```python
from build123d import *

# Parameters (mm, degrees)
F0_W          = 60
F0_H          = 60
F0_R          = 3.5
F1_DEPTH      = 8
F1_DEPTH_BACK = 8
F2_R          = 5.75
F3_DEPTH      = 14
F5_DEPTH      = 60
F8_DEPTH      = 60
F10_W         = 55
F10_H         = 55
F11_DEPTH     = 12


with BuildPart() as f1:
    # F0 (on Top) → F1 (new body, two sides)
    with BuildSketch(Plane.XY) as f1_sk:
        Rectangle(F0_W, F0_H)
        Circle(F0_R, mode=Mode.SUBTRACT)
    extrude(amount=F1_DEPTH)
    extrude(f1_sk.sketch, amount=-F1_DEPTH_BACK)

    # F2 (on face) → F3 (cut)
    with BuildSketch(Plane.XY.offset(8)):
        Circle(F2_R)
    extrude(amount=-F3_DEPTH, mode=Mode.SUBTRACT)

    # F4 (on face) → F5 (join)
    with BuildSketch(Plane(origin=(-30, 0, 0), x_dir=(0, -1, 0), z_dir=(-1, 0, 0))):
        with BuildLine():
            ThreePointArc((-30, 1), (-32.1306623863, 0), (-30, -1))
            Line((-30, -1), (-30, 1))
        make_face()
    extrude(amount=-F5_DEPTH)

    # F6: F1 across plane


with BuildPart() as f1_1:
    add(f1.part)
    add(f1.part.mirror(Plane.XZ))

    # F7 (on face) → F8 (join)
    with BuildSketch(Plane(origin=(0, 30, 0), x_dir=(-1, 0, 0), z_dir=(0, 1, 0))):
        with BuildLine():
            ThreePointArc((30, -1), (32.1306623863, 0), (30, 1))
            Line((30, 1), (30, -1))
        make_face()
    extrude(amount=-F8_DEPTH)

    # F9: F1 across plane


with BuildPart() as f1_2:
    add(f1_1.part)
    add(f1_1.part.mirror(Plane.YZ))

    # F10 (on face) → F11 (cut)
    with BuildSketch(Plane.XY.offset(8)):
        Rectangle(F10_W, F10_H)
    extrude(amount=-F11_DEPTH, mode=Mode.SUBTRACT)


solid = f1_2.part
```
The listing builds one solid part. Answer for the finished solid, in the listing's coordinates (mm). A direction names the side the tool comes from. Give positions to 0.01 mm unless a question says otherwise; leave off trailing zeros. Write each loop counter-clockwise with the first axis right and the second up, starting at its lowest first coordinate (ties: lowest second). Pieces come first, ordered by that corner, then holes. Notation, with made-up numbers: M 6,85.25 L 65,85.25 A10 ccw 65,101.25 Z; hole C -12,14 d1. An arc over 180 degrees is marked long. Write each question's results on one line, items separated by ' | '.
Q1. Consider L1, parallel to X at y = 0, z = -4.75; L2, parallel to Y at x = 2, z = 4.5; L3, parallel to Y at x = 0, z = -7.4. Determine where each line is inside the solid, lowest interval first. Write a range as from..to.
Output values:
L1: -30..-5.75, 5.75..30 | L2: -30..-27.5, 27.5..30 | L3: -30..-3.5, 3.5..30
Q2. Flat-ended cylindrical pins translate along their axes: P1, Ø3, axis at y = -0.5, z = 4.5, coming from the -X side; P2, Ø3, axis at x = 11, z = 4, coming from the -Y side; P3, Ø0.6, axis at y = 31, z = 0.5, coming from the +X side. Find the tip coordinate at first contact, or state that the pin passes through.
Output values:
P1: x = -30 | P2: y = -30 | P3: x = 30
Q3. Section B-B, the plane z = 0 is taken. Write down the section's boundary in (x, y), then the cut area to 3 significant figures.
Output values:
outline: M -32.13,-30 L -30,-30 L -30,-32.13 L 30,-32.13 L 30,-30 L 32.13,-30 L 32.13,30 L 30,30 L 30,32.13 L -30,32.13 L -30,30 L -32.13,30 Z; hole M -27.5,-27.5 L 27.5,-27.5 L 27.5,27.5 L -27.5,27.5 Z | area: 1,090 mm2
Q4. Section D-D, the plane x = -26 is taken. Write down the section's boundary in (y, z).
Output values:
outline: M -30,-8 L 30,-8 L 30,-1 A1.3 ccw long 30,1 L 30,8 L 27.5,8 L 27.5,-4 L -27.5,-4 L -27.5,8 L -30,8 L -30,1 A1.3 ccw long -30,-1 Z
Q5. Section A-A, the plane y = 0 is taken. Write down the section's boundary in (x, z).
Output values:
outline: M -30,-8 L -3.5,-8 L -3.5,-6 L -5.75,-6 L -5.75,-4 L -27.5,-4 L -27.5,8 L -30,8 L -30,1 A1.3 ccw long -30,-1 Z; M 3.5,-8 L 30,-8 L 30,-1 A1.3 ccw long 30,1 L 30,8 L 27.5,8 L 27.5,-4 L 5.75,-4 L 5.75,-6 L 3.5,-6 Z
Q6. For a pull along X with two mould halves and no side action, classify faces 1 (the flat face through (0, 6, -4)), 2 (the cylindrical face through (-32.13, 0.42, -0.04)), 3 (the flat face through (-7, 0, -8)), 4 (the flat face through (30, -31, 0)) as released by +X, released by -X, zero draft, split by the parting line, or undercut.
Output values:
face 1: undercut | face 2: undercut | face 3: zero draft | face 4: released by +X
Q7. A tool of negligible diameter and unlimited length cuts with its end or side. For faces 5 (the flat face through (30, 31, 0)), 6 (the cylindrical face through (-0.75, 5.7, -4.99)), 7 (the cylindrical face through (3.233, -1.341, -6.986)), 8 (the flat face through (-31, 30, 0)), from which of +Z, -Z, +X, -X, +Y, -Y can it reach the whole face along a straight path? Write none if from no direction.
Output values:
face 5: +Z, -Z, +X, +Y | face 6: +Z | face 7: +Z, -Z | face 8: +Z, -Z, -X, +Y
